Solid Edge part; units mm, degrees
sketch "Sketch1" plane through (0, 0, 0) normal (0, -1, 0) x (1, 0, 0)
  line L0 (130, 0) -> (130, 120)
  line L1 (130, 120) -> (0, 120)
  line L2 (0, 120) -> (0, 0)
  line L3 (0, 0) -> (130, 0)
extrude "Protrusion1" add sketch "Sketch1" against normal blind 3
sketch "Sketch2" plane through (66.405, 0, 60) normal (0, -1, 0) x (1, 0, 0)
  line L0 (59.595, 60) -> (59.595, -60)
  line L1 (59.595, -60) -> (63.595, -60)
  line L2 (63.595, -60) -> (63.595, 60)
  line L3 (63.595, 60) -> (59.595, 60)
extrude "Protrusão_Extrudada_2" add sketch "Sketch2" against normal blind 7.0697
sketch "Sketch3" plane through (66.405, 0, 60) normal (0, -1, 0) x (1, 0, 0)
  line L0 (1.595, -11.7379) -> (-26.405, -11.7379)
  line L1 (-26.405, -11.7379) -> (-26.405, -31.7379)
  line L2 (-26.405, -31.7379) -> (1.595, -31.7379)
  line L3 (1.595, -31.7379) -> (1.595, -11.7379)
extrude "Recorte_Extrudado_2" cut sketch "Sketch3" against normal blind 60.6919
Verification items for the finished model (mm, model axes). A direction names the side the tool comes from. Round coordinates to 2 decimals unless told otherwise and drop trailing zeros. Write each loop counter-clockwise with the first axis right and the second up, starting at its lowest first coordinate (ties: lowest second). Pieces come first, ordered by that corner, then holes.
1. Section check D-D on z = 50.5. Enter the section's corners in (x, y).
2. Section check A-A on x = 65. Enter the section's corners in (y, z).
3. Draft check along Z on faces 4 (the flat face through (66, 1, 120)), 5 (the flat face through (126, 5, 61)), 6 (the flat face through (54, 1, 28.262)). Enter one of: +Z half, -Z half, draft (parallel to the pull), parting line (faces both ways), or undercut.
4. Scan lines: L1, parallel to Z at x = 47, y = 1.75; L2, parallel to X at y = 3.75, z = 29.5; L3, parallel to Y at x = 114, z = 58.5. Record each from-to range of solid material in increasing order.
5. Gauge pin test, flat ends, axial feed: P1, Ø3.5, axis at y = 6, z = 56.5, coming from the -X side; P2, Ø1, axis at x = 108, z = 25, coming from the +Y side. Record the tip position at first contact, or that the pin passes through.
6. Access from +Z, -Z, +X, -X, +Y, -Y to the whole of each face (thin tool, end or side, straight path). Record for faces 1 (the flat face through (40, 1, 38)), 2 (the flat face through (64, 3, 61)), 3 (the flat face through (64, 1, 0)).
7. Section check C-C on y = 1.75. Enter the section's corners in (x, z).
8. Section check B-B on z = 38. Enter the section's corners in (x, y), plus the area to 3 significant figures.
Answer:
1. outline: (0, 0) - (130, 0) - (130, 7.07) - (126, 7.07) - (126, 3) - (0, 3) - close
2. outline: (0, 0) - (3, 0) - (3, 28.26) - (0, 28.26) - close; (0, 48.26) - (3, 48.26) - (3, 120) - (0, 120) - close
3. face 4: +Z half
3. face 5: draft
3. face 6: undercut
4. L1: z = 0 to 28.26, 48.26 to 120
4. L2: x = 126 to 130
4. L3: y = 0 to 3
5. P1: stops at x = 126
5. P2: stops at y = 3
6. face 1: +Y, -Y
6. face 2: +Z, -Z, -X, +Y
6. face 3: -Z, +X, -X, +Y, -Y
7. outline: (0, 0) - (130, 0) - (130, 120) - (0, 120) - close; hole (40, 28.26) - (68, 28.26) - (68, 48.26) - (40, 48.26) - close
8. outline: (0, 0) - (40, 0) - (40, 3) - (0, 3) - close; (68, 0) - (130, 0) - (130, 7.07) - (126, 7.07) - (126, 3) - (68, 3) - close
8. area: 322 mm2
